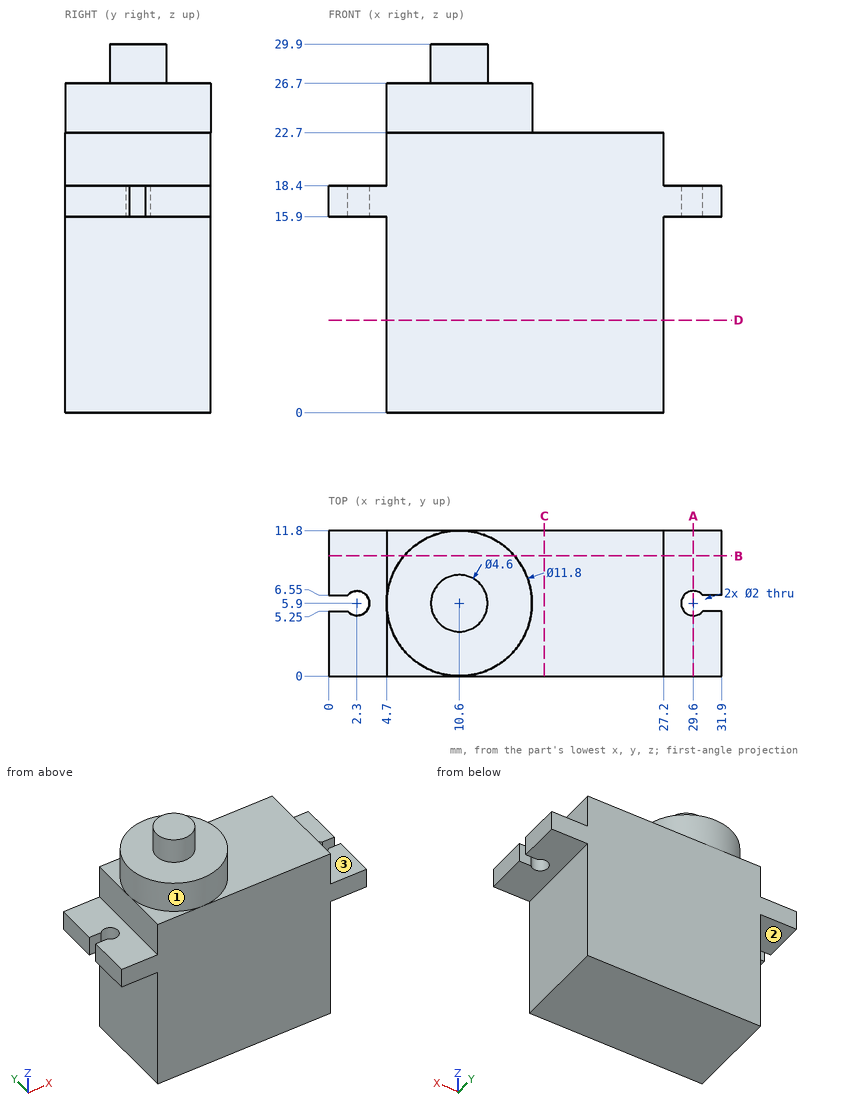
Source: three-view drawing plus pictorial views. Frame: mm from the lowest corner of the part. A direction names the side the tool comes from. Give positions to 0.01 mm unless a question says otherwise; leave off trailing zeros. Write each loop counter-clockwise with the first axis right and the second up, starting at its lowest first coordinate (ties: lowest second). Pieces come first, ordered by that corner, then holes. Notation, with made-up numbers: (-19.75, 39) - (23.25, 39) arc R26 cw to (23.25, 68) - close; hole circle Ø5 at (-16.5, 19.25). An arc over 180 degrees is marked (long way). Write item = value, one per line. Start each with the question number.
1. First-contact query: pin 1 Ø6 at (y, z) = (2, 12) entering from +X; pin 2 Ø6 at (x, y) = (11, 3.5) entering from +Z; pin 3 Ø2 at (x, y) = (26.5, 4.5) entering from +Z; pin 4 Ø4.5 at (x, y) = (7, 9) entering from +Z. Flat tips, straight axial feed; report the tip coordinate or a pass-through.
2. Ray query, L1, parallel to Y at x = 29.6, z = 17.75; L2, parallel to X at y = 5.9, z = 17.25; L3, parallel to Z at x = 4.5, y = 8.5. Return the intervals inside material, ascending.
3. Section query C-C, the plane x = 17.5. Output: boundary loops of the cut face in (y, z), then the cut area to 3 significant figures.
4. Section query D-D, the plane z = 7.5. Output: boundary loops of the cut face in (x, y), then the cut area to 4 significant figures.
5. Access query for the marked faces 1, 2 and 3. Directions: +Z, -Z, +X, -X, +Y, -Y. A direction counts if a zero-diameter tool reaches every point of the face in a straight line with its end or side. Return the directions, or none.
6. Section query A-A, the plane x = 29.6. Output: boundary loops of the cut face in (y, z), then the cut area to 3 significant figures.
7. Section query B-B, the plane y = 9.75. Output: boundary loops of the cut face in (x, z), then the cut area to 3 significant figures.
Check sheet entries:
q1.pin_1 = 27.2
q1.pin_2 = 29.9
q1.pin_3 = 22.7
q1.pin_4 = 26.7
q2.L1 = 0 to 4.9, 6.9 to 11.8
q2.L2 = 3.3 to 28.6
q2.L3 = 15.9 to 18.4
q3.outline = (0, 0) - (11.8, 0) - (11.8, 22.7) - (0, 22.7) - close
q3.area = 268 mm2
q4.outline = (4.7, 0) - (27.2, 0) - (27.2, 11.8) - (4.7, 11.8) - close
q4.area = 265.5 mm2
q5.face_1 = +Z
q5.face_2 = -Z, -X, +Y, -Y
q5.face_3 = +Z, +X, +Y, -Y
q6.outline = (0, 15.9) - (4.9, 15.9) - (4.9, 18.4) - (0, 18.4) - close; (6.9, 15.9) - (11.8, 15.9) - (11.8, 18.4) - (6.9, 18.4) - close
q6.area = 24.5 mm2
q7.outline = (0, 15.9) - (4.7, 15.9) - (4.7, 0) - (27.2, 0) - (27.2, 15.9) - (31.9, 15.9) - (31.9, 18.4) - (27.2, 18.4) - (27.2, 22.7) - (15.07, 22.7) - (15.07, 26.7) - (6.13, 26.7) - (6.13, 22.7) - (4.7, 22.7) - (4.7, 18.4) - (0, 18.4) - close
q7.area = 570 mm2
